Geometry check sheet. Reference: the model listing, model coordinates, mm. A direction names the side the tool comes from. Coordinates: 2 decimals unless noted, no trailing zeros. Loops run counter-clockwise (first coordinate to the right, second up) from the corner with the lowest first, then second, coordinate; pieces in that order, holes last. Notation, with made-up numbers: (30.25, -25) - (88.25, -25) arc R28 ccw to (88.25, -3) - close; hole circle Ø8 at (-3.75, 72.25). An arc over 180 degrees is marked (long way). Write each question's results on one line, items separated by ' | '. Start each with the question number.
(1) Sectioned sample at C-C (y = 4). Enter the section's corners in (x, z), plus the area to 3 significant figures.
(2) Sectioned sample at B-B (x = 0). Enter the section's corners in (y, z), plus the area to 3 significant figures.
(3) Go/stop test with flat-tipped pins: pin 1 Ø5 at (y, z) = (9.5, 3) entering from -X; pin 2 Ø1.5 at (y, z) = (7.5, -2.5) entering from -X. Record where each tip stops, or that it passes through.
(4) Access from +Z, -Z, +X, -X, +Y, -Y to the whole of each face (thin tool, end or side, straight path). Record for faces 1 (the face through (2.44, 4.06, 0.54)), 2 (the face through (0, 16, 6)).
(5) Material ranges on probe 1 along Y at (x, z) = (3.5, -4); probe 2 along Y at (x, z) = (2.5, 1.25); probe 3 along Z at (x, y) = (0, 9.5), recorded low to high.
(6) Sectioned sample at A-A (z = 0). Enter the section's corners in (x, y).
(7) Sectioned sample at D-D (y = 14.25). Enter the section's corners in (x, z), plus the area to 3 significant figures.
from build123d import *

# Parameters (mm, degrees)
SKETCH_2_W          = 2
SKETCH_2_H          = 8
CUT_EXTRUDE_1_DEPTH = 10


with BuildPart() as part:
    # 草图1 → 旋转1 (revolve)
    with BuildSketch(Plane(origin=(0, 0, 0), x_dir=(0, 0, -1), z_dir=(1, 0, 0))):
        Polygon((0, 0), (2.5, 0), (2.5, 8), (3, 8), (3, 14), (6, 14), (6, 17), (0, 17), align=None)
    revolve(axis=Axis((0, 0, 0), (0, 1, 0)))

    # 草图2 → 切除-拉伸1 (cut)
    with BuildSketch(Plane(origin=(0, 17, 0), x_dir=(1, 0, 0), z_dir=(0, 1, 0))):
        with Locations((-6, 0)):
            Rectangle(SKETCH_2_W, SKETCH_2_H)
        with Locations((6, 0)):
            Rectangle(SKETCH_2_W, SKETCH_2_H)
    extrude(amount=-CUT_EXTRUDE_1_DEPTH, mode=Mode.SUBTRACT)


solid = part.part
Outcome:
1) outline: circle Ø5 at (0, 0) | area: 19.6 mm2
2) outline: (0, -2.5) - (8, -2.5) - (8, -3) - (14, -3) - (14, -6) - (17, -6) - (17, 6) - (14, 6) - (14, 3) - (8, 3) - (8, 2.5) - (0, 2.5) - close | area: 112 mm2
3) pin 1: stops at x = -2.96 | pin 2: stops at x = -2.29
4) face 1: -Y | face 2: +Z, +Y, -Y
5) probe 1: y = 14 to 17 | probe 2: y = 8 to 17 | probe 3: z = -3 to 3
6) outline: (-5, 14) - (-3, 14) - (-3, 8) - (-2.5, 8) - (-2.5, 0) - (2.5, 0) - (2.5, 8) - (3, 8) - (3, 14) - (5, 14) - (5, 17) - (-5, 17) - close
7) outline: (-5, -3.32) arc R6 ccw to (5, -3.32) - (5, 3.32) arc R6 ccw to (-5, 3.32) - close | area: 104 mm2
